Design review of the part built by this model. Coordinates are the model's own, in mm. Face numbers are marked on the shaded views. Give positions to 0.01 mm unless a question says otherwise; leave off trailing zeros. Order: outer loops, then holes, each group sorted by start corner. A loop starts at its lowest first (then second) coordinate and runs counter-clockwise, first axis right, second up. Notation, with made-up numbers: (65.25, 47.25) -> (79.25, 47.25) arc R12 ccw to (79.25, 66.25) -> close; hole circle Ø11 at (-9.75, -27). An arc over 180 degrees is marked (long way). Answer in a Markdown table with one row per item. Add a question column.
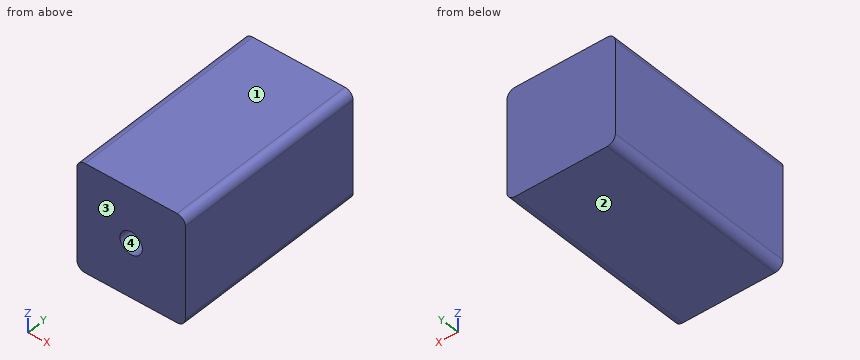
```python
from build123d import *

# Parameters (mm, degrees)
SKETCH_1_W               = 40
SKETCH_1_H               = 72.85
BLOCKEXTRUDE_DEPTH       = 40
FILLET_2_R               = 3
SKETCH_2_R               = 4.15
MOTOR_SHAFT_SOCKET_DEPTH = 26


with BuildPart() as part:
    # 草图1 → BlockExtrude (new body)
    with BuildSketch(Plane.XY):
        with Locations((20, 36.425)):
            Rectangle(SKETCH_1_W, SKETCH_1_H)
    extrude(amount=BLOCKEXTRUDE_DEPTH)

    # Fillet 2
    fillet_2_edges = [part.edges().sort_by_distance(p)[0] for p in [
        (40, 36.425, 40),
        (0, 36.425, 40),
        (40, 36.425, 0),
        (0, 36.425, 0),
    ]]
    fillet(fillet_2_edges, radius=FILLET_2_R)

    # 草图2 → Motor_shaft_socket (cut)
    with BuildSketch(Plane.XZ):
        with Locations(Location((20, 20, 0), (0, 0, 270))):
            Circle(SKETCH_2_R)
    extrude(amount=-MOTOR_SHAFT_SOCKET_DEPTH, mode=Mode.SUBTRACT)


solid = part.part
```
1) Mouldability with a two-part tool opening along Z and no side actions: class the marked faces 1, 2, 3 and 4 as +Z half, -Z half, draft (parallel to the pull), parting line (faces both ways), or undercut.
2) Add section A-A, the plane z = 20. Write out the cut boundary in (x, y), and give its area (3 significant figures).
3) Add section B-B, the plane x = 20. Write out the cut boundary in (y, z), and give its area (3 significant figures).
4) For L1, parallel to X at y = 20, z = 20, list the stretches that pass through material, from the lowest coordinate up.
5) Clearance check with a flat-ended pin moving along its axis: P1, Ø4, axis at x = 19, z = 20.5, coming from the -Y side. State where the tip first meets the part, or that it passes through.
Verdict:
| question | item | result |
|---|---|---|
| 1 | face 1 | +Z half |
| 1 | face 2 | -Z half |
| 1 | face 3 | draft |
| 1 | face 4 | undercut |
| 2 | outline | (0, 0) -> (15.85, 0) -> (15.85, 26) -> (24.15, 26) -> (24.15, 0) -> (40, 0) -> (40, 72.85) -> (0, 72.85) -> close |
| 2 | area | 2,700 mm2 |
| 3 | outline | (0, 0) -> (72.85, 0) -> (72.85, 40) -> (0, 40) -> (0, 24.15) -> (26, 24.15) -> (26, 15.85) -> (0, 15.85) -> close |
| 3 | area | 2,700 mm2 |
| 4 | L1 | x = 0 to 15.85, 24.15 to 40 |
| 5 | P1 | stops at y = 26 |
